```python
from build123d import *

# Parameters (mm, degrees)
SKETCH_W        = 45
SKETCH_H        = 20
SKETCH_R        = 1.6
PAD_DEPTH       = 4
FILLET_R        = 3
SKETCH001_R     = 2.8
POCKET_DEPTH    = 2
POCKET001_DEPTH = 4.001
POCKET002_DEPTH = 2


with BuildPart() as part:
    # Sketch → Pad (new body)
    with BuildSketch(Plane.XY):
        Rectangle(SKETCH_W, SKETCH_H)
        with Locations((-17.186, 0)):
            Circle(SKETCH_R, mode=Mode.SUBTRACT)
        with Locations((17.186, 0)):
            Circle(SKETCH_R, mode=Mode.SUBTRACT)
    extrude(amount=PAD_DEPTH)

    # Fillet
    fillet_edges = [part.edges().sort_by_distance(p)[0] for p in [
        (22.5, 10, 2),
        (22.5, -10, 2),
        (-22.5, -10, 2),
        (-22.5, 10, 2),
    ]]
    fillet(fillet_edges, radius=FILLET_R)

    # Sketch001 (on Face5 of Fillet) → Pocket (cut)
    with BuildSketch(Plane.XY.offset(4)):
        with Locations((-17.186, 0)):
            Circle(SKETCH001_R)
        with Locations((17.186, 0)):
            Circle(SKETCH001_R)
    extrude(amount=-POCKET_DEPTH, mode=Mode.SUBTRACT)

    # Sketch002 (on Face5 of Pocket) → Pocket001 (cut, through all)
    with BuildSketch(Plane.XY.offset(4)):
        with BuildLine():
            ThreePointArc((-17.186, 1.6), (-18.786, 0), (-17.186, -1.6))
            Line((-17.186, -1.6), (-10.5, -1.6))
            ThreePointArc((-10.5, -1.6), (-8.9, 0), (-10.5, 1.6))
            Line((-10.5, 1.6), (-17.186, 1.6))
        make_face()
        with BuildLine():
            ThreePointArc((10.5, 1.6), (8.9, 0), (10.5, -1.6))
            Line((10.5, -1.6), (17.186, -1.6))
            ThreePointArc((17.186, -1.6), (18.786, 0), (17.186, 1.6))
            Line((17.186, 1.6), (10.5, 1.6))
        make_face()
    extrude(amount=-POCKET001_DEPTH, mode=Mode.SUBTRACT)

    # Sketch003 (on Face5 of Pocket001) → Pocket002 (cut)
    with BuildSketch(Plane.XY.offset(4)):
        with BuildLine():
            ThreePointArc((-17.186, 2.8), (-19.986, 0), (-17.186, -2.8))
            Line((-17.186, -2.8), (-10.5, -2.8))
            ThreePointArc((-10.5, -2.8), (-7.7, 0), (-10.5, 2.8))
            Line((-10.5, 2.8), (-17.186, 2.8))
        make_face()
        with BuildLine():
            ThreePointArc((10.5, 2.8), (7.7, 0), (10.5, -2.8))
            Line((10.5, -2.8), (17.186, -2.8))
            ThreePointArc((17.186, -2.8), (19.986, 0), (17.186, 2.8))
            Line((17.186, 2.8), (10.5, 2.8))
        make_face()
    extrude(amount=-POCKET002_DEPTH, mode=Mode.SUBTRACT)


solid = part.part
```
CAD build for the part. Positions are in the model's coordinates, mm. A direction names the side the tool comes from. Round coordinates to 2 decimals unless told otherwise and drop trailing zeros. Loops run counter-clockwise (first coordinate to the right, second up) from the corner with the lowest first, then second, coordinate; pieces in that order, holes last. Notation, with made-up numbers: (20, -14.5) - (60, -14.5) arc R30 cw to (60, 16.5) - close; hole circle Ø8 at (-9.75, 46.5). An arc over 180 degrees is marked (long way). Return JSON: item names as keys, results as strings. Group by question number.
Q1. Band-saw the part on A-A on z = 2.55. Give the cut face in (x, y).
Q2. Two-plate mould, pull along X, no slides. Class faces 4 (the face through (21.6, -9.14, 2.03)), 5 (the face through (0, 10, 2)), 6 (the face through (-18.786, 0.035, 0.986)): +X half, -X half, draft (parallel to the pull), parting line (faces both ways), or undercut.
Q3. Flat gauge pins, fed straight in: pin 1 Ø1.7 at (x, y) = (11, -1) entering from +Z; pin 2 Ø6 at (x, y) = (-15.5, -1) entering from +Z. Where does each tip first touch, or does it go through?
Q4. Band-saw the part on C-C on x = 14. Give the cut face in (y, z), plus the area to 3 significant figures.
Q5. Tool access for faces 1 (the face through (0, -10, 2)), 2 (the face through (-14, 1.6, 1)), 3 (the face through (14, -2, 2)): list every direction of +Z, -Z, +X, -X, +Y, -Y with a clear straight run to the whole face (end or side of a thin tool).
Q6. Band-saw the part on D-D on y = 2.25. Give the cut face in (x, z).
Q7. Drill centre lines: line 1 along Y through (x, z) = (-17, 1.2); line 2 along Y through (x, z) = (-14, 3.65); line 3 along X through (y, z) = (-1.75, 2.1). Where is each one in solid material? Low to high. Write a range as [from, to].
Q8. Band-saw the part on B-B on y = 0. Give the cut face in (x, z), plus the area to 3 significant figures.
Solutions:
{
 "1": {"outline": "(-22.5, -7) arc R3 ccw to (-19.5, -10) - (19.5, -10) arc R3 ccw to (22.5, -7) - (22.5, 7) arc R3 ccw to (19.5, 10) - (-19.5, 10) arc R3 ccw to (-22.5, 7) - close; hole (-17.19, -2.8) - (-10.5, -2.8) arc R2.8 ccw to (-10.5, 2.8) - (-17.19, 2.8) arc R2.8 ccw to start; hole (10.5, -2.8) - (17.19, -2.8) arc R2.8 ccw to (17.19, 2.8) - (10.5, 2.8) arc R2.8 ccw to start"},
 "2": {"face 4": "+X half", "face 5": "draft", "face 6": "undercut"},
 "3": {"pin 1": "stops at z = 2", "pin 2": "stops at z = 4"},
 "4": {"outline": "(-10, 0) - (-1.6, 0) - (-1.6, 2) - (-2.8, 2) - (-2.8, 4) - (-10, 4) - close; (1.6, 0) - (10, 0) - (10, 4) - (2.8, 4) - (2.8, 2) - (1.6, 2) - close", "area": "62.4 mm^2"},
 "5": {"face 1": "+Z, -Z, +X, -X, -Y", "face 2": "+Z, -Z", "face 3": "+Z"},
 "6": {"outline": "(-22.5, 0) - (22.5, 0) - (22.5, 4) - (18.85, 4) - (18.85, 2) - (8.83, 2) - (8.83, 4) - (-8.83, 4) - (-8.83, 2) - (-18.85, 2) - (-18.85, 4) - (-22.5, 4) - close"},
 "7": {"line 1": "y = [-10, -1.6], [1.6, 10]", "line 2": "y = [-10, -2.8], [2.8, 10]", "line 3": "x = [-22.5, -19.37], [-8.31, 8.31], [19.37, 22.5]"},
 "8": {"outline": "(-22.5, 0) - (-18.79, 0) - (-18.79, 2) - (-19.99, 2) - (-19.99, 4) - (-22.5, 4) - close; (-8.9, 0) - (8.9, 0) - (8.9, 2) - (7.7, 2) - (7.7, 4) - (-7.7, 4) - (-7.7, 2) - (-8.9, 2) - close; (18.79, 0) - (22.5, 0) - (22.5, 4) - (19.99, 4) - (19.99, 2) - (18.79, 2) - close", "area": "91.3 mm^2"}
}
